Source: CAD feature listing. Evaluate the final solid. Frame: model axes, mm. Face numbers are marked on the shaded views. A direction names the side the tool comes from. Give positions to 0.01 mm unless a question says otherwise; leave off trailing zeros. Write each loop counter-clockwise with the first axis right and the second up, starting at its lowest first coordinate (ties: lowest second). Pieces come first, ordered by that corner, then holes. Notation, with made-up numbers: (-34.75, 80) -> (20.25, 80) arc R33 ccw to (20.25, 109) -> close; hole circle Ø1 at (-26, -29). An arc over 180 degrees is marked (long way). Use one line per item in the form item = value. Start each with the question number.
(1) Draft query along X for the marked faces 1, 2 and 3. Return one class per face: pulls with the +X half, pulls with the -X half, needs draft (parallel to the pull), parting line crosses it, or undercut.
(2) Material intervals for line 1 along Y through (x, z) = (0, 33); line 2 along Y through (x, z) = (10.5, -31); line 3 along X through (y, z) = (12, -32), sorted ascending. Write a range as from..to.
(3) Cut plane C-C, the plane y = -50.5. Output: boundary loops of the cut face in (x, z).
(4) First-contact query: P1, Ø8, axis at x = -8.5, y = -118.5, coming from the -Z side; P2, Ø10, axis at x = 0, y = 18.75, coming from the -Z side; P3, Ø10, axis at x = 18.5, y = -263.5, coming from the +Z side. Flat tips, straight axial feed; report the tip coordinate or a pass-through.
(5) Cut plane B-B, the plane y = -7. Output: boundary loops of the cut face in (x, z).
(6) Cut plane A-A, the plane x = 11. Output: boundary loops of the cut face in (y, z).
(7) Cut plane D-D, the plane z = 7. Output: boundary loops of the cut face in (x, y), and give its area (3 significant figures).
(8) Set-up query: the marked faces 4, 5, 6, 7 and 8. Return all of +Z, -Z, +X, -X, +Y, -Y with unobstructed straight access to the full face (end or side cutting, diameter ignored); none if empty.
from build123d import *

# Parameters (mm, degrees)
SKETCH1_R           = 28.1
BOSS_EXTRUDE2_DEPTH = 61.3
SKETCH3_R           = 18.6
CUT_EXTRUDE2_DEPTH  = 58.8
SKETCH4_W           = 56.2
SKETCH4_H           = 56.2
BOSS_EXTRUDE3_DEPTH = 56.2
SKETCH5_R           = 16.1
CUT_EXTRUDE4_DEPTH  = 5
SKETCH6_W           = 49.797391422
SKETCH6_H           = 49.779255452
CUT_EXTRUDE5_DEPTH  = 53.7
SKETCH7_R           = 28.1
BOSS_EXTRUDE4_DEPTH = 321.5
CUT_EXTRUDE6_DEPTH  = 10
SKETCH9_R           = 3
CUT_EXTRUDE7_DEPTH  = 1
SKETCH10_R          = 6.025
CUT_EXTRUDE8_DEPTH  = 0.1
SKETCH18_R          = 3.75
CUT_EXTRUDE9_DEPTH  = 100
SKETCH19_R          = 3.75
CUT_EXTRUDE11_DEPTH = 325


with BuildPart() as part:
    # Sketch1 → Boss-Extrude2 (new body)
    with BuildSketch(Plane.XY):
        Circle(SKETCH1_R)
    extrude(amount=BOSS_EXTRUDE2_DEPTH)

    # Sketch3 → Cut-Extrude2 (cut)
    with BuildSketch(Plane.XY.offset(61.3)):
        with Locations((0, -7)):
            Circle(SKETCH3_R)
    extrude(amount=-CUT_EXTRUDE2_DEPTH, mode=Mode.SUBTRACT)

    # Sketch4 → Boss-Extrude3 (add)
    with BuildSketch(Plane(origin=(0, 0, 0), x_dir=(-1, 0, 0), z_dir=(0, 0, -1))):
        Rectangle(SKETCH4_W, SKETCH4_H)
    extrude(amount=BOSS_EXTRUDE3_DEPTH)

    # Sketch5 → Cut-Extrude4 (cut)
    with BuildSketch(Plane.XY.offset(2.5)):
        with Locations((0, -7)):
            Circle(SKETCH5_R)
    extrude(amount=-CUT_EXTRUDE4_DEPTH, mode=Mode.SUBTRACT)

    # Sketch6 → Cut-Extrude5 (cut)
    with BuildSketch(Plane(origin=(0, 0, -56.2), x_dir=(-1, 0, 0), z_dir=(0, 0, -1))):
        Rectangle(SKETCH6_W, SKETCH6_H)
    extrude(amount=-CUT_EXTRUDE5_DEPTH, mode=Mode.SUBTRACT)

    # Sketch7 → Boss-Extrude4 (add)
    with BuildSketch(Plane(origin=(0, -28.1, 0), x_dir=(-1, 0, 0), z_dir=(0, -1, 0))):
        with Locations(Location((0, 28.1, 0), (0, 0, 90))):
            Circle(SKETCH7_R)
    extrude(amount=BOSS_EXTRUDE4_DEPTH)

    # Sketch8 → Cut-Extrude6 (cut)
    with BuildSketch(Plane(origin=(0, -349.6, 0), x_dir=(-1, 0, 0), z_dir=(0, -1, 0))):
        with BuildLine():
            Line((-1.658312395, 25.832078896), (1.658312395, 25.832078896))
            ThreePointArc((1.658312395, 25.832078896), (3, 28.332078896), (1.658312395, 30.832078896))
            Line((1.658312395, 30.832078896), (-1.658312395, 30.832078896))
            ThreePointArc((-1.658312395, 30.832078896), (-3, 28.332078896), (-1.658312395, 25.832078896))
        make_face()
    extrude(amount=-CUT_EXTRUDE6_DEPTH, mode=Mode.SUBTRACT)

    # Sketch9 → Cut-Extrude7 (cut)
    with BuildSketch(Plane(origin=(0, -349.6, 0), x_dir=(-1, 0, 0), z_dir=(0, -1, 0))):
        with Locations(Location((0, 28.332078896, 0), (0, 0, 90))):
            Circle(SKETCH9_R)
    extrude(amount=-CUT_EXTRUDE7_DEPTH, mode=Mode.SUBTRACT)

    # Sketch10 → Cut-Extrude8 (cut)
    with BuildSketch(Plane(origin=(0, -349.6, 0), x_dir=(-1, 0, 0), z_dir=(0, -1, 0))):
        with Locations(Location((0, 28.332078896, 0), (0, 0, 90))):
            Circle(SKETCH10_R)
    extrude(amount=-CUT_EXTRUDE8_DEPTH, mode=Mode.SUBTRACT)

    # Cut-Sweep4: sweep along a path in Sketch15
    with BuildLine(Plane(origin=(0, -349.6, 0), x_dir=(-1, 0, 0), z_dir=(0, -1, 0))) as cut_sweep4_path:
        ThreePointArc((15, 28.332078896), (0, 43.332078896), (-15, 28.332078896))
    # 3DSketch2 → Cut-Sweep4 (sweep, cut)
    with BuildSketch(Plane(origin=(-15, -349.6, -28.332078896), x_dir=(-0.022748965612757834, 0.999741208795331, 0), z_dir=(0, 0, 1))):
        Polygon((0, 0), (0.170617242, 7.498059066), (329.685319661, 0), (329.514702419, -7.498059066), align=None)
    sweep(path=cut_sweep4_path.line, mode=Mode.SUBTRACT)

    # Sketch18 → Cut-Extrude9 (cut)
    with BuildSketch(Plane.XY.offset(61.3)):
        with Locations((0, 18.75)):
            Circle(SKETCH18_R)
    extrude(amount=-CUT_EXTRUDE9_DEPTH, mode=Mode.SUBTRACT)

    # Sketch19 → Cut-Extrude11 (cut)
    with BuildSketch(Plane(origin=(0, -349.6, 0), x_dir=(-1, 0, 0), z_dir=(0, -1, 0))):
        with Locations((-18.75, 28.332078896)):
            Circle(SKETCH19_R)
        with Locations((18.75, 28.332078896)):
            Circle(SKETCH19_R)
    extrude(amount=-CUT_EXTRUDE11_DEPTH, mode=Mode.SUBTRACT)


solid = part.part
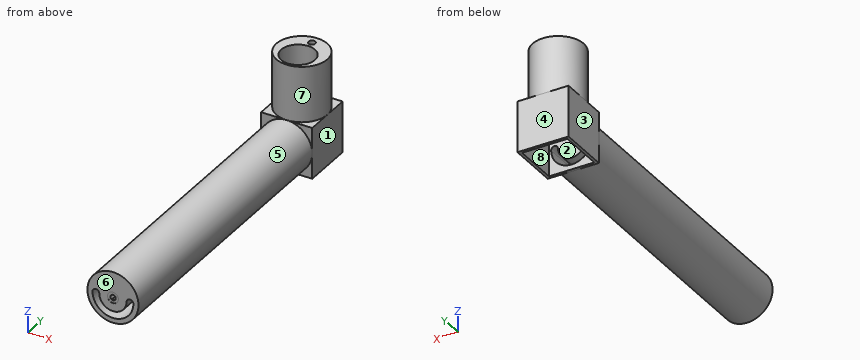
Geometry says:
q1.face_1 = pulls with the +X half
q1.face_2 = undercut
q1.face_3 = pulls with the -X half
q2.line_1 = -28.1..-25.6, 11.6..15, 22.5..28.1
q2.line_2 = -349.6..-24.89, 24.89..28.1
q2.line_3 = -28.1..-24.9, 24.9..28.1
q3.outline = circle Ø56.2 at (0, -28.1); hole (-22.5, -28.33) arc R22.5 ccw to (22.5, -28.33) arc R3.75 ccw to (15, -28.33) arc R15 cw to (-15, -28.33) arc R3.75 ccw to start
q4.P1 = -55.84
q4.P2 = -2.5
q4.P3 = -3.46
q5.outline = (-28.1, -56.2) -> (-24.9, -56.2) -> (-24.9, -2.5) -> (-16.1, -2.5) -> (-16.1, 2.5) -> (-18.6, 2.5) -> (-18.6, 61.3) -> (-27.21, 61.3) -> (-27.21, 0) -> (-28.1, 0) -> close; (16.1, -2.5) -> (24.9, -2.5) -> (24.9, -56.2) -> (28.1, -56.2) -> (28.1, 0) -> (27.21, 0) -> (27.21, 61.3) -> (18.6, 61.3) -> (18.6, 2.5) -> (16.1, 2.5) -> close
q6.outline = (-349.6, -53.96) -> (-28.1, -53.96) -> (-28.1, -56.2) -> (-24.89, -56.2) -> (-24.89, -47.96) -> (-349.6, -47.96) -> close; (-349.6, -38.53) -> (-24.89, -38.53) -> (-24.89, -2.5) -> (-18.76, -2.5) -> (-18.76, 2.5) -> (-22, 2.5) -> (-22, 61.3) -> (-25.86, 61.3) -> (-25.86, 0) -> (-28.1, 0) -> (-28.1, -2.24) -> (-349.6, -2.24) -> close; (4.76, -2.5) -> (24.89, -2.5) -> (24.89, -56.2) -> (28.1, -56.2) -> (28.1, 0) -> (25.86, 0) -> (25.86, 61.3) -> (8, 61.3) -> (8, 2.5) -> (4.76, 2.5) -> close
q7.outline = circle Ø56.2 at (0, 0); hole circle Ø37.2 at (0, -7); hole circle Ø7.5 at (0, 18.75)
q7.area = 1,350 mm^2
q8.face_4 = +Z, -Z, +X, -X, +Y
q8.face_5 = -Y
q8.face_6 = +Z, -Z, +X, -X, -Y
q8.face_7 = +Z
q8.face_8 = -Z
